Geometry check sheet. Reference: the model listing, model coordinates, mm. A direction names the side the tool comes from. Coordinates: 2 decimals unless noted, no trailing zeros. Write each loop counter-clockwise with the first axis right and the second up, starting at its lowest first coordinate (ties: lowest second). Pieces come first, ordered by that corner, then holes. Notation, with made-up numbers: (45.5, -34) -> (59.5, -34) arc R17 ccw to (59.5, -18) -> close; hole circle Ø2 at (-7, 65). An arc over 180 degrees is marked (long way). One line per question, with ' | ' between items.
from build123d import *

# Parameters (mm, degrees)
F0_W      = 50.8
F0_H      = 50.8
F0_R      = 12.7
F1_DEPTH  = 50.8
F2_R      = 13.682638
F3_DEPTH  = 25.4
F3_FACE_R = 13.682638
F4_DEPTH  = 25.4
F5_W      = 25.4
F5_H      = 25.56793
F6_DEPTH  = 25.4
F7_R      = 12.7
F8_DEPTH  = 25.4


with BuildPart() as f1:
    # F0 (on Front) → F1 (new body)
    with BuildSketch(Plane.XZ):
        with Locations((-25.4, 25.4)):
            Rectangle(F0_W, F0_H)
        with Locations((-26.229173, 23.804629)):
            Circle(F0_R, mode=Mode.SUBTRACT)
        with Locations((-26.229173, 23.804629)):
            Circle(F0_R)
    extrude(amount=F1_DEPTH)

    # F2 (on face) → F3 (cut)
    with BuildSketch(Plane(origin=(0, 0, 0), x_dir=(-1, 0, 0), z_dir=(0, 1, 0))):
        with Locations((25.127107, 25.4)):
            Circle(F2_R)
    extrude(amount=-F3_DEPTH, mode=Mode.SUBTRACT)

    # F3_face (on face) → F4 (cut)
    with BuildSketch(Plane(origin=(-25.127107, -25.4, 25.4), x_dir=(-1, 0, 0), z_dir=(0, 1, 0))):
        Circle(F3_FACE_R)
    extrude(amount=-F4_DEPTH, mode=Mode.SUBTRACT)

    # F5 (on face) → F6 (join)
    with BuildSketch(Plane(origin=(-50.8, 0, 0), x_dir=(0, -1, 0), z_dir=(-1, 0, 0))):
        with Locations((26.313143, 23.804629)):
            Rectangle(F5_W, F5_H)
    extrude(amount=F6_DEPTH)

    # F7 (on face) → F8 (join)
    with BuildSketch(Plane.XY.offset(50.8)):
        with Locations((-27.772067, -25.4)):
            Circle(F7_R)
    extrude(amount=F8_DEPTH)


solid = f1.part
1. Cross-section at C-C on x = -34. Record the boundary of the cut face in (y, z), and give its area (3 significant figures).
Worked answers:
outline: (-50.8, 0) -> (0, 0) -> (0, 14.98) -> (-50.8, 14.98) -> close; (-50.8, 35.82) -> (0, 35.82) -> (0, 50.8) -> (-14.33, 50.8) -> (-14.33, 76.2) -> (-36.47, 76.2) -> (-36.47, 50.8) -> (-50.8, 50.8) -> close | area: 2,080 mm²
2. Cross-section at D-D on y = -3. Record the boundary of the cut face in (x, z).
Worked answers:
outline: (-50.8, 0) -> (0, 0) -> (0, 50.8) -> (-50.8, 50.8) -> close; hole circle Ø27.37 at (-25.13, 25.4)
3. Go/stop test with flat-tipped pins: P1, Ø1, axis at x = -36, y = -7, coming from the +Z side; P2, Ø12.5, axis at x = -58.5, z = 20.5, coming from the +Y side; P3, Ø12, axis at y = -39.5, z = 57.5, coming from the +X side; P4, Ø8, axis at x = -46, z = 31, coming from the +Y side. Record where each tip stops, or that it passes through.
Worked answers:
P1: z = 50.8 | P2: y = -13.61 | P3: x = -17.99 | P4: y = 0
4. Tool access check on faces 1 (the face through (-63, -39.013, 24)), 2 (the face through (-16.04, -30.26, 63.32)), 3 (the face through (-63, -26, 36.589)), 4 (the face through (-63, -13.613, 24)), 5 (the face through (-14, -50.8, 14)). Record the directions out of +Z, -Z, +X, -X, +Y, -Y that give a thin tool (end or side, any length) a straight path to the whole face; none if there is none.
Worked answers:
face 1: +Z, -Z, -X, -Y | face 2: +Z | face 3: +Z, -X, +Y, -Y | face 4: +Z, -Z, -X, +Y | face 5: +Z, -Z, +X, -X, -Y
5. Cross-section at A-A on z = 25.4. Record the boundary of the cut face in (x, y).
Worked answers:
outline: (-76.2, -39.01) -> (-50.8, -39.01) -> (-50.8, -50.8) -> (-38.81, -50.8) -> (-38.81, 0) -> (-50.8, 0) -> (-50.8, -13.61) -> (-76.2, -13.61) -> close; (-11.44, -50.8) -> (0, -50.8) -> (0, 0) -> (-11.44, 0) -> close
6. Material ranges on line 1 (Z direction, x = -25, y = -37); line 2 (Z direction, x = -25.5, y = -49); line 3 (X direction, y = -20, z = 25), recorded low to high. Write a range as from..to.
Worked answers:
line 1: 0..11.72, 39.08..76.2 | line 2: 0..11.72, 39.08..50.8 | line 3: -76.2..-38.8, -11.45..0
7. Mould release check, pull along X, two halves, no side actions. Record for faces 6 (the face through (-76.2, -26, 24)), 7 (the face through (-22.161, -25.044, 12.043)), 8 (the face through (0, -25, 25)), 9 (the face through (-63, -26, 11.021)): released by +X, released by -X, zero draft, split by the parting line, or undercut.
Worked answers:
face 6: released by -X | face 7: undercut | face 8: released by +X | face 9: zero draft
8. Cross-section at B-B on y = -25.4. Record the boundary of the cut face in (x, z).
Worked answers:
outline: (-76.2, 11.02) -> (-50.8, 11.02) -> (-50.8, 0) -> (0, 0) -> (0, 50.8) -> (-15.07, 50.8) -> (-15.07, 76.2) -> (-40.47, 76.2) -> (-40.47, 50.8) -> (-50.8, 50.8) -> (-50.8, 36.59) -> (-76.2, 36.59) -> close; hole circle Ø27.37 at (-25.13, 25.4)
